Autodesk Inventor part; units mm, degrees
ref_plane "YZ Plane" through (0, 0, 0) normal (1, 0, 0) x (0, 1, 0)
ref_plane "XZ Plane" through (0, 0, 0) normal (0, 1, 0) x (-1, 0, 0)
ref_plane "XY Plane" through (0, 0, 0) normal (0, 0, 1) x (1, 0, 0)
sketch "Sketch1" plane through (0, 0, 0) normal (0, 1, 0) x (-1, 0, 0)
  line L0 (0, 290.198) -> (0, -290.198) construction
  line L1 (98.4779, 0) -> (-98.4779, 0) construction
  arc A0 (-441.1, 0) -> (-250, -363.4133) centre (0, 0) ccw
  line L2 (-441.1, 0) -> (-441.1, 400)
  line L3 (-441.1, 400) -> (-500, 400)
  line L4 (-500, 400) -> (-500, -363.4133)
  line L5 (-250, -363.4133) -> (-500, -363.4133)
  dimension "d0" = 500
  dimension "d1" = 400
  dimension "d3" = 441.1
  dimension "d5" = 363.4133
extrude "Extrusion1" add sketch "Sketch1" along normal blind 5
sketch "Sketch2" plane through (0, 0, 0) normal (0, -1, 0) x (1, 0, 0)
  line L0 (441.1, 400) -> (500, 400)
  line L1 (441.1, 0) -> (441.1, 400)
  line L2 (0, 0) -> (467.2725, -59.9302) construction
  line L3 (0, 0) -> (442.392, -161.9398) construction
  line L4 (0, 0) -> (395.535, -255.9048) construction
  line L5 (0, 0) -> (329.0291, -337.1573) construction
  line L6 (471.1, 255) -> (471.1, 360) construction
  line L7 (471.1, 255) -> (471.1, 150) construction
  line L8 (471.1, 150) -> (471.1, 45) construction
  line L9 (500, 400) -> (500, -363.4133) construction
  line L10 (471.1, 45) -> (467.2725, -59.9302) construction
  line L11 (467.2725, -59.9302) -> (442.392, -161.9398) construction
  line L12 (442.392, -161.9398) -> (395.535, -255.9048) construction
  line L13 (395.535, -255.9048) -> (329.0291, -337.1573) construction
  point P0 (470.55, 400)
  dimension "d8" = 40
  dimension "d9" = 30
  dimension "d10" = 471.1
  dimension "d15" = 105
hole "Hole1" at (471.1, 0, 360) at (471.1, 0, 255) at (471.1, 0, 150) at (471.1, 0, 45) at (467.2725, 0, -59.9302) at (442.392, 0, -161.9398) at (395.535, 0, -255.9048) at (329.0291, 0, -337.1573) direction (0, 1, 0) diameter 5 end through all
properties part number "boundaryHalf1V1"
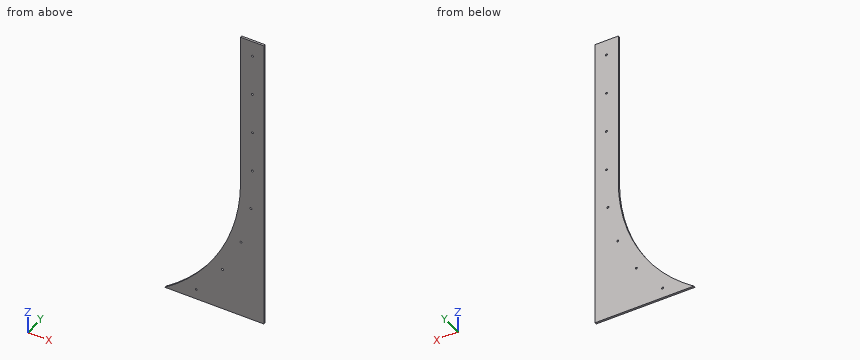
Could you check a few things on this model? Use its own coordinates, in mm. Coordinates: 2 decimals unless noted, no trailing zeros. Order: outer loops, then holes, each group sorted by start corner. A loop starts at its lowest first (then second) coordinate and runs counter-clockwise, first axis right, second up.
Q1. Please list where these lines run through material, in increasing order: L1, parallel to Z at x = 471.1, y = 1.9; L2, parallel to X at y = 4.45, z = 136; L3, parallel to X at y = 3.5, z = 150.
Q2. Suppose I cut it at A-A on y = 2.15. Give the number of separate pieces and of enclosed holes in the cut face, and give its area (3 significant figures).
Q3. Suppose I cut it at C-C on z = -269. Please give me the cut outline in (x, y).
Q4. Suppose I cut it at B-B on z = 185. Please give me the cut outline in (x, y).
Q5. Will this pin go through, and if not, where does the flat tip stop? pin 1 (6 mm diameter, centred on x = 471.1, z = 255, fed in from +Y).
Answer:
1. L1: z = -363.41 to 42.5, 47.5 to 147.5, 152.5 to 252.5, 257.5 to 357.5, 362.5 to 400
1. L2: x = 441.1 to 500
1. L3: x = 441.1 to 468.6, 473.6 to 500
2. separate pieces: 1
2. enclosed holes: 8
2. area: 65,500 mm2
3. outline: (349.58, 0) - (500, 0) - (500, 5) - (349.58, 5) - close
4. outline: (441.1, 0) - (500, 0) - (500, 5) - (441.1, 5) - close
5. pin 1: stops at y = 5
